```python
from build123d import *

# Parameters (mm, degrees)
ESQUISSE1_W              = 280
ESQUISSE1_H              = 210
BOSS_EXTRU_1_DEPTH       = 5
ESQUISSE2_R              = 3
ESQUISSE2_R_2            = 1.5
ESQUISSE2_R_3            = 8
ESQUISSE2_R_4            = 14
ESQUISSE2_R_5            = 10
ESQUISSE2_W              = 52
ESQUISSE2_H              = 78
ENL_V_MAT_EXTRU_1_DEPTH  = 351.035712464
ESQUISSE5_R              = 1.5
ENL_V_MAT_EXTRU_3_DEPTH  = 351.035712464
ESQUISSE6_W              = 280
ESQUISSE6_H              = 93
BOSS_EXTRU_4_DEPTH       = 5
ESQUISSE7_R              = 1.499999999
ENL_V_MAT_EXTRU_4_DEPTH  = 351.035712464
ESQUISSE8_R              = 1.499999999
ENL_V_MAT_EXTRU_5_DEPTH  = 351.035712464
ESQUISSE9_R              = 1.5
ENL_V_MAT_EXTRU_6_DEPTH  = 351.035712464
ESQUISSE14_R             = 23
ESQUISSE14_R_2           = 1.5
ENL_V_MAT_EXTRU_11_DEPTH = 351.035712464


with BuildPart() as part:
    # Esquisse1 → Boss.-Extru.1 (new body)
    with BuildSketch(Plane.XY):
        with Locations((140, 105)):
            Rectangle(ESQUISSE1_W, ESQUISSE1_H)
    extrude(amount=BOSS_EXTRU_1_DEPTH)

    # Esquisse2 → Enlèv. mat.-Extru.1 (cut, through all)
    with BuildSketch(Plane.XY):
        with Locations((270, 190)):
            Circle(ESQUISSE2_R)
        with Locations((10, 190)):
            Circle(ESQUISSE2_R)
        with Locations((10, 20)):
            Circle(ESQUISSE2_R)
        with Locations((270, 20)):
            Circle(ESQUISSE2_R)
        with Locations((187, 168)):
            Circle(ESQUISSE2_R_2)
        with Locations((187, 72)):
            Circle(ESQUISSE2_R_2)
        with Locations((91.5, 128)):
            Circle(ESQUISSE2_R_2)
        with Locations((27, 128)):
            Circle(ESQUISSE2_R_2)
        with Locations((92, 40)):
            Circle(ESQUISSE2_R_2)
        with Locations((26, 40)):
            Circle(ESQUISSE2_R_2)
        with Locations((15, 45)):
            Circle(ESQUISSE2_R_3)
        with Locations((146.093717203, 173)):
            Circle(ESQUISSE2_R_4)
        with Locations((232.477054828, 60.19739042)):
            Circle(ESQUISSE2_R_5)
        with Locations((272.5, 103)):
            Circle(ESQUISSE2_R_2)
        with Locations((272.5, 135)):
            Circle(ESQUISSE2_R_2)
        with Locations((59, 84)):
            Rectangle(ESQUISSE2_W, ESQUISSE2_H)
        Polygon((137.113248654, 63.5), (134.226497308, 58.5), (137.113248654, 53.5), (142.886751346, 53.5), (145.773502692, 58.5), (142.886751346, 63.5), align=None)
    extrude(amount=ENL_V_MAT_EXTRU_1_DEPTH, mode=Mode.SUBTRACT)

    # Esquisse5 → Enlèv. mat.-Extru.3 (cut, through all)
    with BuildSketch(Plane(origin=(0, 0, 0), x_dir=(-1, 0, 0), z_dir=(0, 0, -1))):
        with Locations((-93, 179.4)):
            Circle(ESQUISSE5_R)
        with Locations((-93, 199.4)):
            Circle(ESQUISSE5_R)
        with Locations((-187, 199.4)):
            Circle(ESQUISSE5_R)
        with Locations((-187, 179.4)):
            Circle(ESQUISSE5_R)
    extrude(amount=-ENL_V_MAT_EXTRU_3_DEPTH, mode=Mode.SUBTRACT)

    # Esquisse6 → Boss.-Extru.4 (add)
    with BuildSketch(Plane(origin=(0, 0, 0), x_dir=(-1, 0, 0), z_dir=(0, 0, -1))):
        with Locations((-140, -46.5)):
            Rectangle(ESQUISSE6_W, ESQUISSE6_H)
    extrude(amount=-BOSS_EXTRU_4_DEPTH)

    # Esquisse7 → Enlèv. mat.-Extru.4 (cut, through all)
    with BuildSketch(Plane(origin=(0, 0, 0), x_dir=(-1, 0, 0), z_dir=(0, 0, -1))):
        with Locations((-42.785302694, -27.055649919)):
            Circle(ESQUISSE7_R)
        with Locations((-42.773346208, -63.039616064)):
            Circle(ESQUISSE7_R)
    extrude(amount=-ENL_V_MAT_EXTRU_4_DEPTH, mode=Mode.SUBTRACT)

    # Esquisse8 → Enlèv. mat.-Extru.5 (cut, through all)
    with BuildSketch(Plane(origin=(0, 0, 0), x_dir=(-1, 0, 0), z_dir=(0, 0, -1))):
        with Locations((-245.944892864, -62.344865672)):
            Circle(ESQUISSE8_R)
        with Locations((-245.944892864, -26.360897541)):
            Circle(ESQUISSE8_R)
    extrude(amount=-ENL_V_MAT_EXTRU_5_DEPTH, mode=Mode.SUBTRACT)

    # Esquisse9 → Enlèv. mat.-Extru.6 (cut, through all)
    with BuildSketch(Plane(origin=(0, 0, 0), x_dir=(-1, 0, 0), z_dir=(0, 0, -1))):
        with Locations((-93, -62.4)):
            Circle(ESQUISSE9_R)
        with Locations((-93, -82.4)):
            Circle(ESQUISSE9_R)
        with Locations((-187, -82.4)):
            Circle(ESQUISSE9_R)
        with Locations((-187, -62.4)):
            Circle(ESQUISSE9_R)
    extrude(amount=-ENL_V_MAT_EXTRU_6_DEPTH, mode=Mode.SUBTRACT)

    # Esquisse14 → Enlèv. mat.-Extru.11 (cut, through all)
    with BuildSketch(Plane(origin=(0, 0, 0), x_dir=(-1, 0, 0), z_dir=(0, 0, -1))):
        with Locations((-54.48265068, 163.570126578)):
            Circle(ESQUISSE14_R)
        with Locations((-54.649127802, 193.569664664)):
            Circle(ESQUISSE14_R_2)
        with Locations((-54.316173557, 133.570588492)):
            Circle(ESQUISSE14_R_2)
    extrude(amount=-ENL_V_MAT_EXTRU_11_DEPTH, mode=Mode.SUBTRACT)


solid = part.part
```
Work out the finished part from the listing and answer in its coordinate system (mm). Coordinates: 2 decimals unless noted, no trailing zeros. Write each loop counter-clockwise with the first axis right and the second up, starting at its lowest first coordinate (ties: lowest second). Pieces come first, ordered by that corner, then holes.
Q1. A cutting plane is placed at B-B, the plane y = 148. Give the vertices of the cut face in (x, z).
Q2. Determine the mould class of faces 1 (the face through (13.959, 52.932, 2.465)), 2 (the face through (173, 61, 0)) for opening direction X: released by +X, released by -X, zero draft, split by the parting line, or undercut.
Q3. A cutting plane is placed at A-A, the plane y = 89.5. Give the vertices of the cut face in (x, z), then the cut area to 3 significant figures.
Q4. Find the intervals of material crossed by line 1 (X direction, y = 190, z = 4.75); line 2 (X direction, y = -82.4, z = 3.9); line 3 (Y direction, x = 270, z = 2.05), in increasing order.
Q5. Each of these flat-tipped pins is pushed along its axis until it touches: pin 1 Ø3 at (x, y) = (219, -41) entering from -Z; pin 2 Ø2.5 at (x, y) = (54.32, 133.57) entering from -Z. Where does it stop, or does it pass through?
Q6. A cutting plane is placed at C-C, the plane z = 1.15. State how many separate pieces and enclosed holes the cut face has, then the cut area to 3 significant figures.
Findings below:
1. outline: (0, 0) - (37.55, 0) - (37.55, 5) - (0, 5) - close; (71.41, 0) - (280, 0) - (280, 5) - (71.41, 5) - close
2. face 1: undercut
2. face 2: zero draft
3. outline: (0, 0) - (33, 0) - (33, 5) - (0, 5) - close; (85, 0) - (280, 0) - (280, 5) - (85, 5) - close
3. area: 1,140 mm2
4. line 1: x = 0 to 7, 13 to 267, 273 to 280
4. line 2: x = 0 to 91.5, 94.5 to 185.5, 188.5 to 280
4. line 3: y = -93 to 17, 23 to 187, 193 to 210
5. pin 1: stops at z = 0
5. pin 2: passes through
6. separate pieces: 1
6. enclosed holes: 32
6. area: 77,600 mm2
